The model under review builds one solid part; all positions refer to its coordinate system, in mm. Face numbers are marked on the shaded views. A direction names the side the tool comes from. Give positions to 0.01 mm unless a question says otherwise; leave off trailing zeros. Order: outer loops, then holes, each group sorted by start corner. A loop starts at its lowest first (then second) coordinate and runs counter-clockwise, first axis right, second up. Notation, with made-up numbers: (70, 80) - (105, 80) arc R22 cw to (105, 101) - close; hole circle Ø3 at (69, -14). An arc over 180 degrees is marked (long way). Use CSV: the item, a comma, the result in double quotes. Start each with the question number.
1. To check wall thickness, follow line 1 (X direction, y = 452, z = 278); line 2 (Y direction, x = 75, z = 226.5); line 3 (Z direction, x = 61, y = 450). State the ranges of each line that lie inside material, in increasing order. Write a range as [from, to].
2. Take a section at B-B, the plane x = 84. State the section outline as (y, z) points, then the cut area to 3 significant figures.
3. For pin 1 (4 mm diameter, centred on y = 454, z = 218.5, fed in from +X); pin 2 (5.5 mm diameter, centred on y = 450, z = 197, fed in from -X); pin 3 (2 mm diameter, centred on x = 66, y = 458.5, fed in from +Z), all flat-tipped, find the tip position at first contact; note any pin that passes through.
4. Take a section at C-C, the plane z = 157.5. State the section outline as (x, y) points.
5. Take a section at A-A, the plane z = 263.5. State the section outline as (x, y) points, then the cut area to 3 significant figures.
6. Machinability: for the marked faces 1 and 2, which of the approach directions +Z, -Z, +X, -X, +Y, -Y give a long, thin tool a straight path to every point of the face, cutting with its end or side? Answer none if there is none.
```python
from build123d import *

# Parameters (mm, degrees)
PAD_DEPTH    = 5
SKETCH001_W  = 39
SKETCH001_H  = 12.348814
PAD001_DEPTH = 5
FILLET_R     = 2
FILLET001_R  = 2


with BuildPart() as part:
    # Sketch (on Face5 of Binder) → Pad (new body)
    with BuildSketch(Plane(origin=(8e-06, 448.000007, 1.5e-05), x_dir=(-1, 0, 0), z_dir=(0, 1, 0))):
        with BuildLine():
            ThreePointArc((-76.138322, 296.60498), (-78.259642, 295.726301), (-79.138322, 293.60498))
            Line((-79.138322, 140.123388), (-79.138322, 293.60498))
            ThreePointArc((-79.138322, 140.123388), (-78.259642, 138.002067), (-76.138322, 137.123388))
            Line((-67.138322, 137.123388), (-76.138322, 137.123388))
            ThreePointArc((-67.138322, 137.123388), (-65.017001, 138.002067), (-64.138322, 140.123388))
            Line((-64.138322, 293.60498), (-64.138322, 140.123388))
            ThreePointArc((-64.138322, 293.60498), (-65.017001, 295.726301), (-67.138322, 296.60498))
            Line((-76.138322, 296.60498), (-67.138322, 296.60498))
        make_face()
        with BuildLine():
            ThreePointArc((-70.488322, 289.068935), (-72.138322, 290.718935), (-73.788322, 289.068935))
            Line((-73.788322, 289.068935), (-73.788322, 239.181824))
            ThreePointArc((-73.788322, 239.181824), (-72.138322, 237.531824), (-70.488322, 239.181824))
            Line((-70.488322, 239.181824), (-70.488322, 289.068935))
        make_face(mode=Mode.SUBTRACT)
        with BuildLine():
            ThreePointArc((-70.488322, 233.068934), (-72.138322, 234.718934), (-73.788322, 233.068934))
            Line((-73.788322, 233.068934), (-73.788322, 183.181823))
            ThreePointArc((-73.788322, 183.181823), (-72.138322, 181.531823), (-70.488322, 183.181823))
            Line((-70.488322, 183.181823), (-70.488322, 233.068934))
        make_face(mode=Mode.SUBTRACT)
    extrude(amount=PAD_DEPTH)

    # Sketch001 (on Face4 of Pad) → Pad001 (join)
    with BuildSketch(Plane(origin=(0, -5e-06, 137.123388), x_dir=(1, 0, 0), z_dir=(0, 0, -1))):
        with Locations((71.638329, -454.174413)):
            Rectangle(SKETCH001_W, SKETCH001_H)
    extrude(amount=-PAD001_DEPTH)

    # Fillet
    fillet_edges = [part.edges().sort_by_distance(p)[0] for p in [
        (52.138329, 460.348815, 139.623403),
        (91.138329, 460.348815, 139.623403),
        (52.138329, 448.000002, 139.623403),
        (91.138329, 448.000002, 139.623403),
    ]]
    fillet(fillet_edges, radius=FILLET_R)

    # Fillet001
    fillet001_edges = [part.edges().sort_by_distance(p)[0] for p in [
        (79.13833, 450.500001, 142.123403),
        (64.13833, 450.500002, 142.123403),
    ]]
    fillet(fillet001_edges, radius=FILLET001_R)


solid = part.part
```
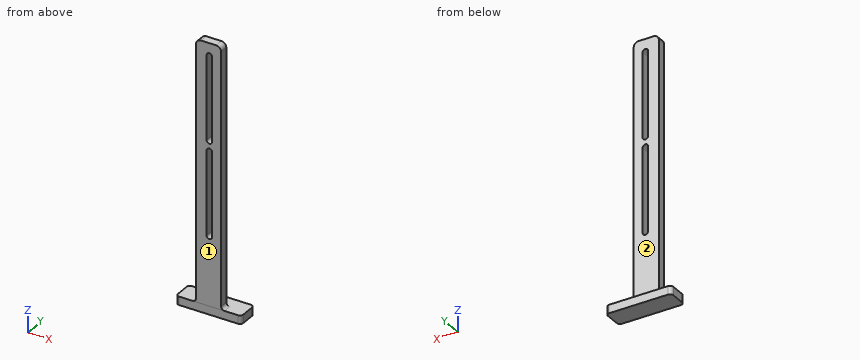
Determined:
1,line 1,"x = [64.14, 70.49], [73.79, 79.14]"
1,line 2,"y = [448, 453]"
1,line 3,"z = [137.12, 142.12]"
2,outline,"(448, 137.12) - (460.35, 137.12) - (460.35, 142.12) - (448, 142.12) - close"
2,area,"61.7 mm²"
3,pin 1,"stops at x = 79.14"
3,pin 2,"stops at x = 64.14"
3,pin 3,"stops at z = 142.12"
4,outline,"(64.14, 448) - (79.14, 448) - (79.14, 453) - (64.14, 453) - close"
5,outline,"(64.14, 448) - (70.49, 448) - (70.49, 453) - (64.14, 453) - close; (73.79, 448) - (79.14, 448) - (79.14, 453) - (73.79, 453) - close"
5,area,"58.5 mm²"
6,face 1,"+Z, -Z, +X, -X, -Y"
6,face 2,"+Z, +X, -X, +Y"
